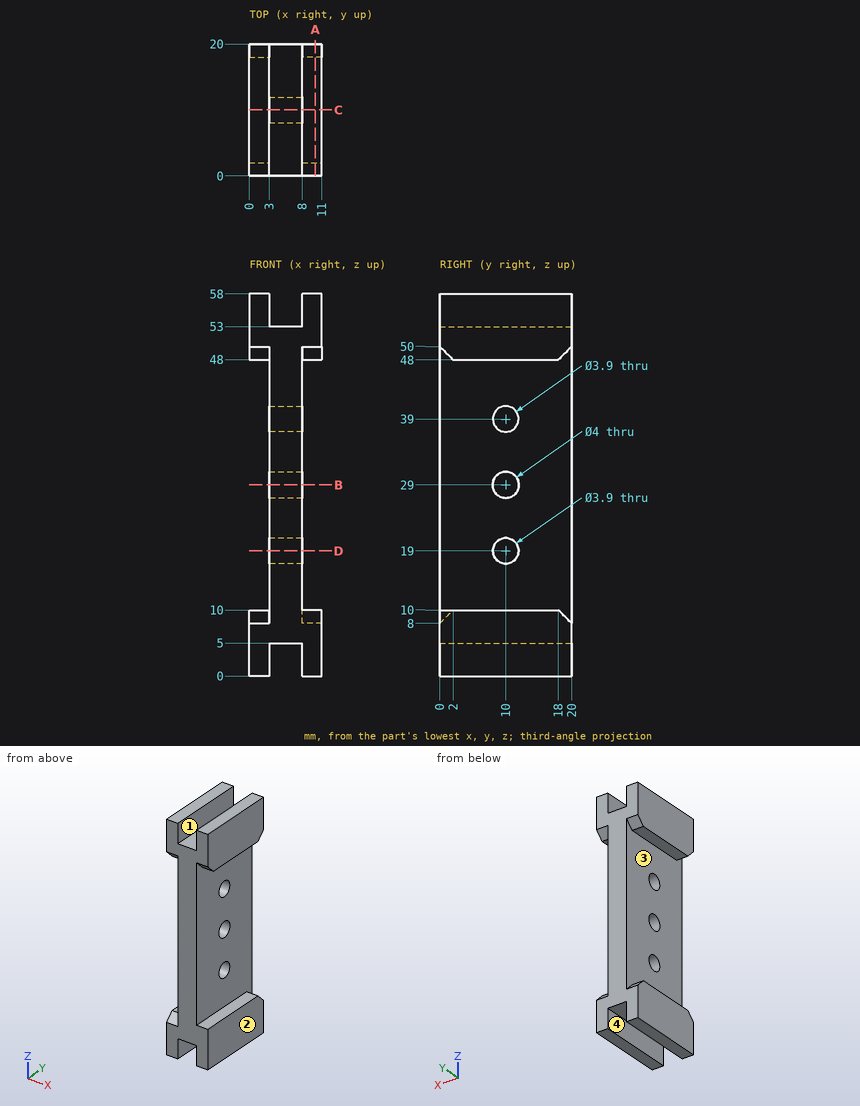
Design review of the part shown in the three views and the two pictorial views. Dimensions are in mm from the part's minimum x, y and z. A direction names the side the tool comes from. Give positions to 0.01 mm unless a question says otherwise; leave off trailing zeros. Loops run counter-clockwise (first coordinate to the right, second up) from the corner with the lowest first, then second, coordinate; pieces in that order, holes last. Notation, with made-up numbers: (82, 62) -> (141, 62) arc R7 ccw to (141, 66) -> close; hole circle Ø10 at (5, 43). An arc over 180 degrees is marked (long way). Write each question's results on one line, items separated by ' | '.
Q1. Take a section at C-C, the plane y = 10. Give the number of separate pieces and of enclosed holes in the cut face, plus the area to 3 significant figures.
Reply:
separate pieces: 4 | enclosed holes: 0 | area: 301 mm²
Q2. For pin 1 Ø4 at (x, y) = (5.5, 7.5) entering from +Z; pin 2 Ø2 at (y, z) = (11, 27) entering from +X; pin 3 Ø3.5 at (y, z) = (10, 19) entering from -X; pin 4 Ø6 at (y, z) = (5.5, 24.5) entering from -X, all flat-tipped, find the tip position at first contact; note any pin that passes through.
Reply:
pin 1: stops at z = 53 | pin 2: stops at x = 8 | pin 3: passes through | pin 4: stops at x = 3
Q3. Machinability: for the marked faces 1 and 2, which of the approach directions +Z, -Z, +X, -X, +Y, -Y give a long, thin tool a straight path to every point of the face, cutting with its end or side? Answer none if there is none.
Reply:
face 1: +Z, +Y, -Y | face 2: +Z, -Z, +X, +Y, -Y
Q4. The part is to be moulded in two halves that separate along Z. For the marked faces 3 and 4, say which applies: +Z half, -Z half, draft (parallel to the pull), parting line (faces both ways), or undercut.
Reply:
face 3: undercut | face 4: draft
Q5. Wall thickness on L1, parallel to Z at x = 9.5, y = 11.25; L2, parallel to Y at x = 6.05, z = 39; L3, parallel to X at y = 18.75, z = 53.5: over which ranges is each line inside the solid? List them lowest first.
Reply:
L1: z = 0 to 10, 48 to 58 | L2: y = 0 to 8.05, 11.95 to 20 | L3: x = 0 to 3, 8 to 11
Q6. Take a section at A-A, the plane x = 10. Write out the cut boundary in (y, z), plus the area to 3 significant figures.
Reply:
outline: (0, 0) -> (20, 0) -> (20, 8) -> (18, 10) -> (0, 10) -> close; (0, 50) -> (2, 48) -> (18, 48) -> (20, 50) -> (20, 58) -> (0, 58) -> close | area: 394 mm²
Q7. Take a section at B-B, the plane z = 29. Write out the cut boundary in (x, y), plus the area to 3 significant figures.
Reply:
outline: (3, 0) -> (8, 0) -> (8, 8) -> (3, 8) -> close; (3, 12) -> (8, 12) -> (8, 20) -> (3, 20) -> close | area: 80.0 mm²
Q8. Take a section at D-D, the plane z = 19. Write out the cut boundary in (x, y).
Reply:
outline: (3, 0) -> (8, 0) -> (8, 8.05) -> (3, 8.05) -> close; (3, 11.95) -> (8, 11.95) -> (8, 20) -> (3, 20) -> close
